Study the drawing (mm; zero at the part's minimum x, y, z) and answer. A direction names the side the tool comes from. Give positions to 0.01 mm unless a question says otherwise; leave off trailing zeros. Order: outer loops, then holes, each group sorted by start corner. A loop starts at its lowest first (then second) coordinate and runs counter-clockwise, first axis right, second up. Notation, with made-up numbers: (-29, 62) - (-24, 62) arc R10 cw to (-24, 73) - close; hole circle Ø3 at (29, 27). An arc over 180 degrees is marked (long way). Write each question's results on one line, items separated by ' | '. Start each with the question number.
1. Section D-D (x = 7.5) is taken. Give the vertices of the cut face in (y, z).
2. Determine the mould class of the marked faces 1, 2 and 3 for opening direction X: released by +X, released by -X, zero draft, split by the parting line, or undercut.
3. Section A-A (z = 7.5) is taken. Give the vertices of the cut face in (x, y).
4. Section C-C (y = 13) is taken. State how many separate pieces and enclosed holes the cut face has, and give its area (3 significant figures).
5. Which of the six approach directions +Z, -Z, +X, -X, +Y, -Y give full straight-line access (tool end or side, diameter ignored) to the marked faces 4 and 5?
6. Section B-B (x = 42.5) is taken. Give the vertices of the cut face in (y, z) (1 decimal), and give its area (3 significant figures).
7. Flat-ended cylindrical pins translate along their axes: pin 1 (4 mm diameter, centred on x = 29.5, z = 40, fed in from -Y); pin 2 (3 mm diameter, centred on x = 7.5, z = 7.5, fed in from +Y); pin 3 (6 mm diameter, centred on x = 40.5, y = 13.5, fed in from -Z); pin 4 (5 mm diameter, centred on y = 3.5, z = 46, fed in from -X). Find the tip coordinate at first contact, or state that the pin passes through.
8. Find the intervals of material crossed by L1, parallel to Z at x = 40, y = 9.25 (1 decimal); L2, parallel to Z at x = 7.5, y = 12.4 (1 decimal); L3, parallel to X at y = 8.75, z = 32.5 (1 decimal), in increasing order.
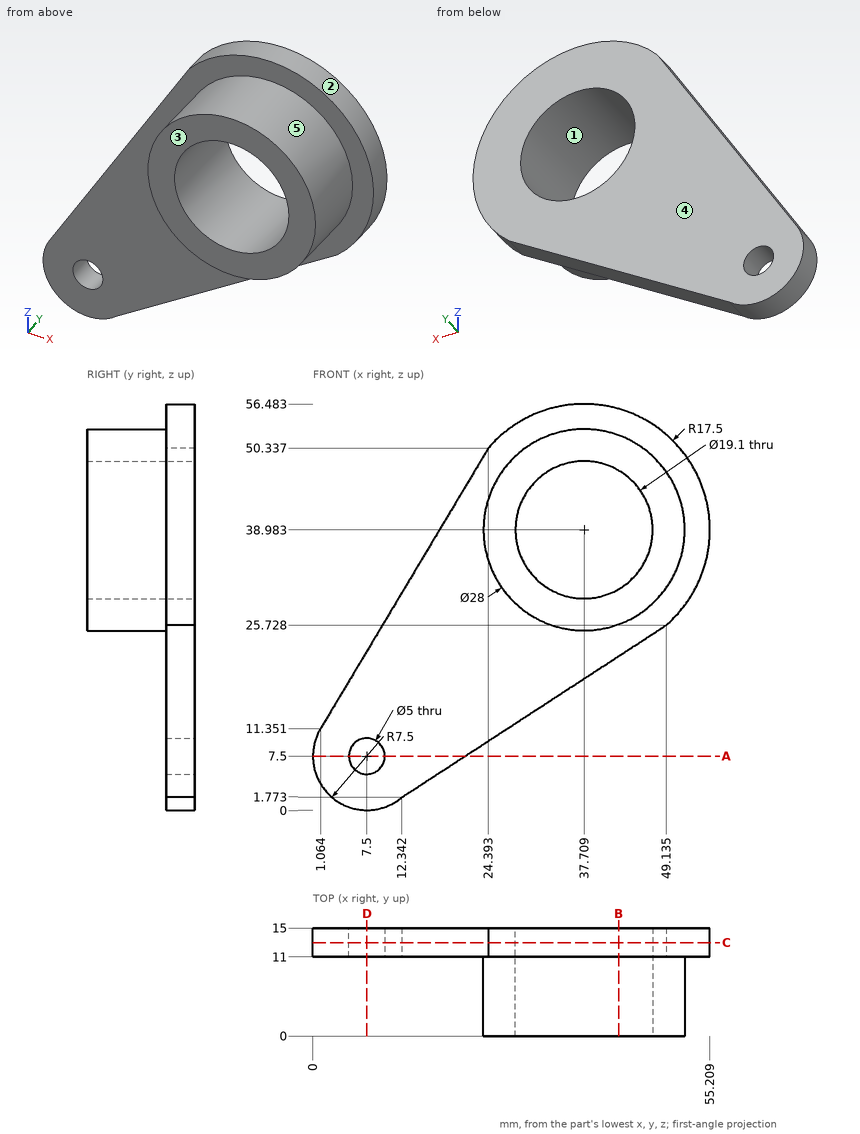
Reported:
1) outline: (11, 0) - (15, 0) - (15, 5) - (11, 5) - close; (11, 10) - (15, 10) - (15, 22.11) - (11, 22.11) - close
2) face 1: undercut | face 2: split by the parting line | face 3: zero draft
3) outline: (0, 11) - (5, 11) - (5, 15) - (0, 15) - close; (10, 11) - (21.14, 11) - (21.14, 15) - (10, 15) - close
4) separate pieces: 1 | enclosed holes: 2 | area: 1,370 mm²
5) face 4: +Z, -Z, +X, -X, +Y | face 5: -Y
6) outline: (0, 25.8) - (11, 25.8) - (11, 21.4) - (15, 21.4) - (15, 30.7) - (0, 30.7) - close; (0, 47.2) - (15, 47.2) - (15, 55.8) - (11, 55.8) - (11, 52.1) - (0, 52.1) - close | area: 179 mm²
7) pin 1: y = 0 | pin 2: through | pin 3: z = 18.15 | pin 4: x = 24.46
8) L1: 25.2 to 29.7, 48.3 to 52.8 | L2: 0 to 5, 10 to 22.1 | L3: 25.3 to 30.7, 44.7 to 50.1
